Build history of the part. All positions in model axes, mm. Face numbers are marked on the shaded views. A direction names the side the tool comes from. Coordinates: 2 decimals unless noted, no trailing zeros. Write each loop counter-clockwise with the first axis right and the second up, starting at its lowest first coordinate (ties: lowest second). Pieces come first, ordered by that corner, then holes.
Autodesk Inventor part; units mm, degrees
ref_plane "Plan YZ" through (0, 0, 0) normal (1, 0, 0) x (0, 1, 0)
ref_plane "Plan XZ" through (0, 0, 0) normal (0, 1, 0) x (-1, 0, 0)
ref_plane "Plan XY" through (0, 0, 0) normal (0, 0, 1) x (1, 0, 0)
sketch "Esquisse1" plane through (0, 0, 0) normal (0, 0, 1) x (1, 0, 0)
  line L0 (0, 0) -> (5, 0)
  line L1 (5, 0) -> (5, 5)
  line L2 (5, 5) -> (4.5, 5)
  line L3 (4.5, 5) -> (4.5, 10)
  line L4 (4.5, 10) -> (0.5, 10)
  line L5 (0.5, 10) -> (0.5, 5)
  line L6 (0.5, 5) -> (0, 5)
  line L7 (0, 5) -> (0, 0)
  dimension "d0" = 5
  dimension "d1" = 5
  dimension "d2" = 5
  dimension "d3" = 4
extrude "Extrusion1" add sketch "Esquisse1" along normal blind 1.25
sketch "Esquisse6" plane through (0, 0, 1.25) normal (0, 0, 1) x (1, 0, 0)
  line L0 (1.5, 0) -> (3.5, 0)
  line L1 (3.5, 0) -> (3.5, 10)
  line L2 (3.5, 10) -> (1.5, 10)
  line L3 (1.5, 10) -> (1.5, 0)
  line L4 (4.5, 10) -> (0.5, 10)
  line L5 (0, 0) -> (5, 0)
  line L6 (4.5, 5) -> (3.5, 5) construction
  line L7 (0.5, 5) -> (1.5, 5) construction
  dimension "d6" = 2
extrude "Extrusion2" add sketch "Esquisse6" along normal blind 0.375 and the other way blind 1.625
sketch "Esquisse7" plane through (3.5, 0, 1.25) normal (1, 0, 0) x (0, 0, -1)
  line L0 (0, 10) -> (-0.375, 10)
  line L1 (-0.375, 10) -> (-0.375, 8.5)
  line L2 (-0.375, 8.5) -> (0, 10)
  line L3 (1.25, 10) -> (1.625, 8.5)
  line L4 (1.625, 8.5) -> (1.625, 10)
  line L5 (1.625, 10) -> (1.25, 10)
  point P0 (1.25, 0)
  dimension "d11" = 1.5
  dimension "d12" = 1.5
extrude "Extrusion3" cut sketch "Esquisse7" against normal blind 2
sketch "Esquisse8" plane through (0, 0, 0) normal (0, 0, -1) x (-1, 0, 0)
  line L0 (-4.5, 9.5) -> (-4, 10)
  line L1 (-4, 10) -> (-4.5, 10)
  line L2 (-4.5, 10) -> (-4.5, 9.5)
  line L3 (-1, 10) -> (-0.5, 9.5)
  line L4 (-0.5, 9.5) -> (-0.5, 10)
  line L5 (-0.5, 10) -> (-1, 10)
  point P0 (0, 0)
  point P1 (-0.5, 10)
  dimension "d15" = 0.5
extrude "Extrusion4" cut sketch "Esquisse8" against normal blind 1.25
equation "\"d1\" = d0"
equation "\"d2\" = d1"
equation "\"d12\" = d11"
properties part number "P1704_009_slider" material "."
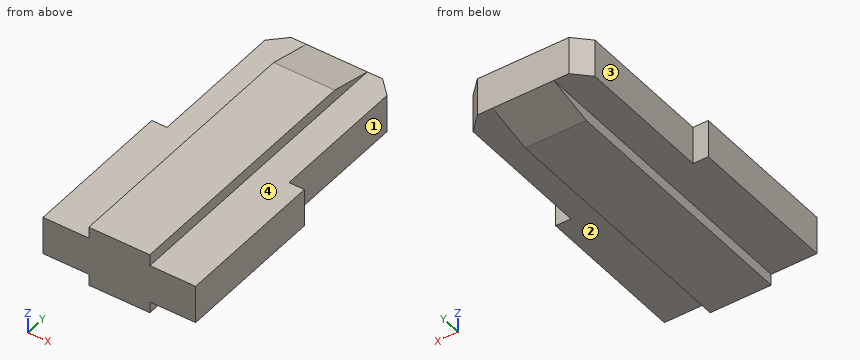
1. Flat gauge pins, fed straight in: pin 1 (1 mm diameter, centred on x = 4.5, y = 4.5, fed in from +Z); pin 2 (1.6 mm diameter, centred on x = 4.5, y = 3, fed in from -Z). Where does each tip first touch, or does it go through?
Computed values:
pin 1: stops at z = 1.25
pin 2: stops at z = 0
2. Saw through at D-D on y = 1.75. List the corners of the cut face in (x, z) (3 decimals).
Computed values:
outline: (0, 0) - (1.5, 0) - (1.5, -0.375) - (3.5, -0.375) - (3.5, 0) - (5, 0) - (5, 1.25) - (3.5, 1.25) - (3.5, 1.625) - (1.5, 1.625) - (1.5, 1.25) - (0, 1.25) - close
3. Probe line 1 along X through (y, z) = (2, 1.5); line 2 along Y through (x, z) = (0.3, 0.2); line 3 along Z through (x, y) = (3.7, 9.5). List the from-to ranges inside material, lowest first.
Computed values:
line 1: x = 1.5 to 3.5
line 2: y = 0 to 5
line 3: z = 0 to 1.25
4. Saw through at B-B on y = 5.5. List the corners of the cut face in (x, z) (3 decimals).
Computed values:
outline: (0.5, 0) - (1.5, 0) - (1.5, -0.375) - (3.5, -0.375) - (3.5, 0) - (4.5, 0) - (4.5, 1.25) - (3.5, 1.25) - (3.5, 1.625) - (1.5, 1.625) - (1.5, 1.25) - (0.5, 1.25) - close
5. Saw through at A-A on z = 0.6. List the corners of the cut face in (x, y).
Computed values:
outline: (0, 0) - (5, 0) - (5, 5) - (4.5, 5) - (4.5, 9.5) - (4, 10) - (1, 10) - (0.5, 9.5) - (0.5, 5) - (0, 5) - close
6. 3-axis set-ups, long thin cutter, end or side, ignore diameter. For the marked faces 1, 2, 3 and 4: which of +Z, -Z, +X, -X, +Y, -Y reach the whole face in a straight line?
Computed values:
face 1: +Z, -Z, +X, +Y
face 2: -Z, +X, +Y, -Y
face 3: +Z, -Z, -X, +Y
face 4: +Z, +X, +Y, -Y
7. Saw through at C-C on x = 2.6. List the corners of the cut face in (y, z) (3 decimals), plus the area to 3 significant figures.
Computed values:
outline: (0, -0.375) - (8.5, -0.375) - (10, 0) - (10, 1.25) - (8.5, 1.625) - (0, 1.625) - close
area: 19.4 mm2
